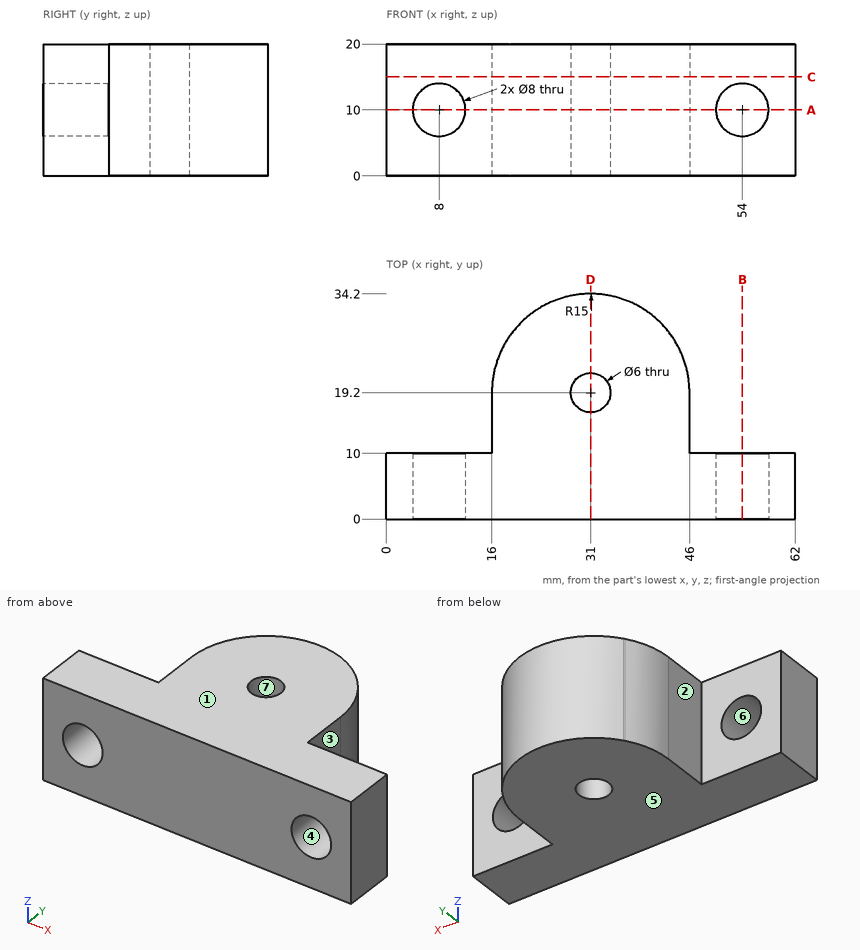
Could you check a few things on this drawing? It's one solid part, dimensions in mm from its lowest x, y, z. A direction names the side the tool comes from. Coordinates: 2 decimals unless noted, no trailing zeros. Order: outer loops, then holes, each group sorted by start corner. A loop starts at its lowest first (then second) coordinate and runs counter-clockwise, first axis right, second up.
1. If we section it at C-C (z = 15): Please give me the cut outline in (x, y).
2. If we section it at A-A (z = 10): Please give me the cut outline in (x, y).
3. If we section it at B-B (x = 54): Please give me the cut outline in (y, z), then the cut area to 3 significant figures.
4. Thinking about a two-plate mould opening in Z: for the marked faces 4, 5, 6 and 7, which applies, +Z half, -Z half, draft (parallel to the pull), parting line (faces both ways), or undercut?
5. I need wall thicknesses on line 1 (Z direction, x = 54, y = 6.5); line 2 (X direction, y = 3, z = 12.5); line 3 (Y direction, x = 31, z = 13). Which ranges of each line are inside material? Lowest first, please.
6. For the marked faces 1, 2 and 3, which set-ups out of +Z, -Z, +X, -X, +Y, -Y let a thin tool reach every point of the face, with its end or its side?
7. If we section it at D-D (x = 31): Please give me the cut outline in (y, z).
8. I'm going to push flat-ended pins straight in: pin 1 (12 mm diameter, centred on x = 16, y = 7.5, fed in from -Z); pin 2 (7 mm diameter, centred on x = 54, z = 10, fed in from -Y); pin 3 (4.5 mm diameter, centred on y = 16, z = 6.5, fed in from -X); pin 4 (6 mm diameter, centred on y = 17.5, z = 10, fed in from +X). Where does each tip first touch, or does it pass through?
Entries:
1. outline: (0, 0) - (62, 0) - (62, 10) - (46, 10) - (46, 19.2) arc R15 ccw to (16, 19.2) - (16, 10) - (0, 10) - close; hole circle Ø6 at (31, 19.2)
2. outline: (0, 0) - (4, 0) - (4, 10) - (0, 10) - close; (12, 0) - (50, 0) - (50, 10) - (46, 10) - (46, 19.2) arc R15 ccw to (16, 19.2) - (16, 10) - (12, 10) - close; (58, 0) - (62, 0) - (62, 10) - (58, 10) - close; hole circle Ø6 at (31, 19.2)
3. outline: (0, 0) - (10, 0) - (10, 6) - (0, 6) - close; (0, 14) - (10, 14) - (10, 20) - (0, 20) - close
3. area: 120 mm2
4. face 4: undercut
4. face 5: -Z half
4. face 6: undercut
4. face 7: draft
5. line 1: z = 0 to 6, 14 to 20
5. line 2: x = 0 to 4.88, 11.12 to 50.88, 57.12 to 62
5. line 3: y = 0 to 16.2, 22.2 to 34.2
6. face 1: +Z, +X, -X, +Y, -Y
6. face 2: +Z, -Z, -X, +Y
6. face 3: +Z, -Z, +X, +Y
7. outline: (0, 0) - (16.2, 0) - (16.2, 20) - (0, 20) - close; (22.2, 0) - (34.2, 0) - (34.2, 20) - (22.2, 20) - close
8. pin 1: stops at z = 0
8. pin 2: passes through
8. pin 3: stops at x = 16
8. pin 4: stops at x = 46
